Can you work these out from the model? Positions are in its coordinate system, mm. A direction names the side the tool comes from. Round coordinates to 2 decimals unless told otherwise and drop trailing zeros. Loops run counter-clockwise (first coordinate to the right, second up) from the corner with the lowest first, then second, coordinate; pieces in that order, holes last.
(1) Will these pins go through, and if not, where does the flat tip stop? pin 1 Ø6 at (x, y) = (6, 13.5) entering from -Z; pin 2 Ø6 at (x, y) = (-13.5, -14.5) entering from +Z.
(2) Which directions (+Z, -Z, +X, -X, +Y, -Y) give clear straight access to the entire face, cutting with the end or side of a thin tool? Please do faces 4 (the face through (0, 0, 1.5)), 5 (the face through (2.343, 17.847, 0.493)).
(3) If I drill on line 1 along Y through (x, z) = (0, 0.85); line 2 along X through (y, z) = (9, 0.2); line 3 along Y through (x, z) = (13, 0.4) (3 decimals), over which ranges is the centre line in solid material (lowest first)?
(4) I want a section at C-C on z = 0.65. Write out the boundary of the cut face in (x, y).
(5) Thinking about a two-plate mould opening in X: for faces 1 (the face through (7, -17, 0)), 2 (the face through (18.409, 5.797, 0.645)), 3 (the face through (0, 0, 1)), which applies, released by +X, released by -X, zero draft, split by the parting line, or undercut?
(6) I want a section at A-A on y = 0. Write out the boundary of the cut face in (x, z), plus the area to 3 significant figures.
from build123d import *

# Parameters (mm, degrees)
ESQUISSE1_R             = 19.3
BOSS_EXTRU_1_DEPTH      = 1.5
ESQUISSE3_R             = 18
ENL_V_MAT_EXTRU_2_DEPTH = 1
CONG_1_R                = 0.5
CONG_2_R                = 0.3


with BuildPart() as part:
    # Esquisse1 → Boss.-Extru.1 (new body)
    with BuildSketch(Plane.XY):
        Circle(ESQUISSE1_R)
    extrude(amount=BOSS_EXTRU_1_DEPTH)

    # Esquisse3 → Enlèv. mat.-Extru.2 (cut)
    with BuildSketch(Plane(origin=(0, 0, 0), x_dir=(-1, 0, 0), z_dir=(0, 0, -1))):
        Circle(ESQUISSE3_R)
    extrude(amount=-ENL_V_MAT_EXTRU_2_DEPTH, mode=Mode.SUBTRACT)

    # Congé1
    cong_1_edges = [part.edges().sort_by_distance(p)[0] for p in [
        (-19.3, 0, 1.5),
    ]]
    fillet(cong_1_edges, radius=CONG_1_R)

    # Congé2
    cong_2_edges = [part.edges().sort_by_distance(p)[0] for p in [
        (-19.3, 0, 0),
    ]]
    fillet(cong_2_edges, radius=CONG_2_R)


solid = part.part
Filled sheet:
1. pin 1: stops at z = 1
1. pin 2: stops at z = 1.5
2. face 4: +Z, +X, -X, +Y, -Y
2. face 5: -Z
3. line 1: y = -19.3 to -18, 18 to 19.3
3. line 2: x = -17.05 to -15.59, 15.59 to 17.05
3. line 3: y = -14.265 to -12.45, 12.45 to 14.265
4. outline: circle Ø38.6 at (0, 0); hole circle Ø36 at (0, 0)
5. face 1: zero draft
5. face 2: split by the parting line
5. face 3: undercut
6. outline: (-19.3, 0.3) arc R0.3 ccw to (-19, 0) - (-18, 0) - (-18, 1) - (18, 1) - (18, 0) - (19, 0) arc R0.3 ccw to (19.3, 0.3) - (19.3, 1) arc R0.5 ccw to (18.8, 1.5) - (-18.8, 1.5) arc R0.5 ccw to (-19.3, 1) - close
6. area: 21.8 mm2
